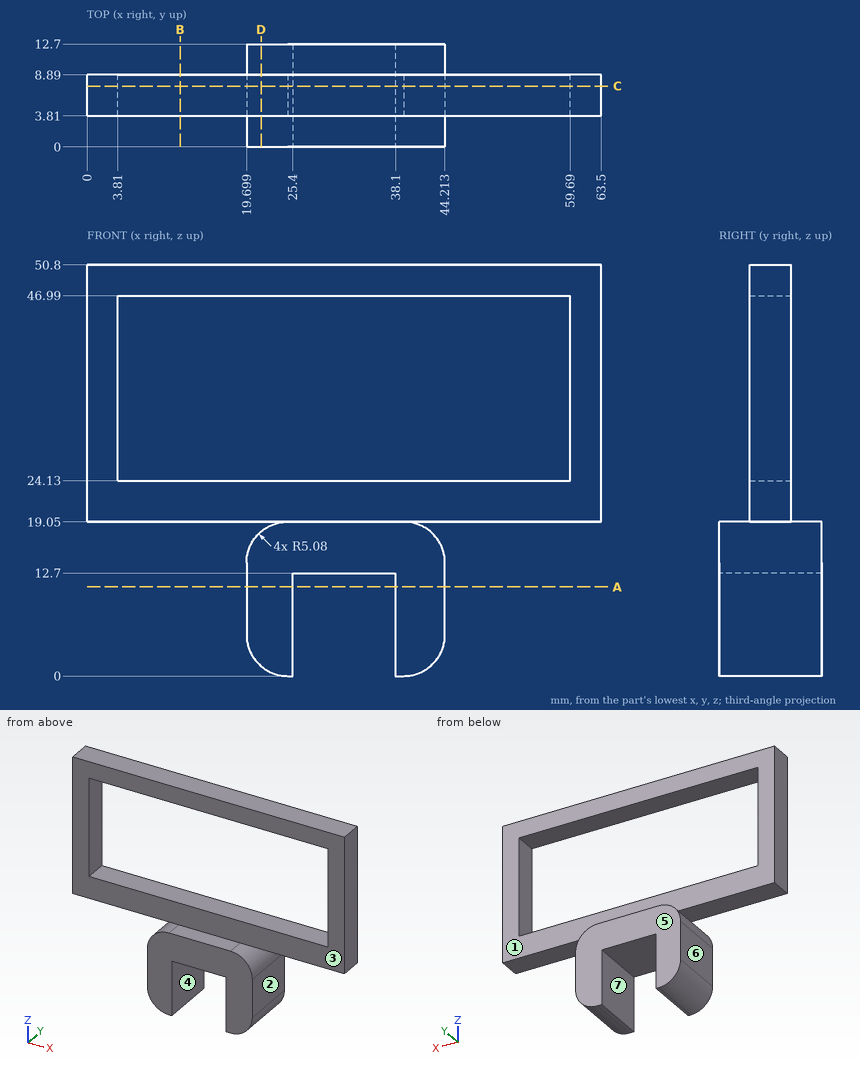
Answer from the drawing. Dimensions are ordinates in mm from the lowest x, y and z of the part. A direction names the side the tool comes from. Give positions to 0.01 mm unless a question says otherwise; leave off trailing zeros. Order: outer loops, then holes, each group sorted by start corner. A loop starts at its lowest first (then second) coordinate and runs counter-clockwise, first axis right, second up. Notation, with made-up numbers: (88.25, 5) -> (98.25, 5) arc R26 ccw to (98.25, 19) -> close; hole circle Ø11 at (10.25, 58). An arc over 180 degrees is marked (long way). Answer as a JSON object with one key per item and string values. Group by question number.
1. Flat-ended cylindrical pins translate along their axes: pin 1 Ø3 at (x, z) = (49.5, 44.5) entering from +Y (3 decimals); pin 2 Ø4 at (x, y) = (22.5, 6) entering from -Z; pin 3 Ø2 at (y, z) = (2, 9) entering from +X; pin 4 Ø4 at (y, z) = (6.5, 3.5) entering from -X. Find the tip coordinate at first contact, or state that the pin passes through.
2. Section B-B on x = 11.5 is taken. Determine the outline of the cut face in (y, z).
3. Section C-C on y = 7.5 is taken. Determine the outline of the cut face in (x, z).
4. Consider line 1 along Z through (x, y) = (54.5, 4); line 2 along X through (y, z) = (8.25, 33); line 3 along X through (y, z) = (1.5, 12). Determine where each line is inside the solid, lowest interval first. Write a range as [from, to].
5. Section A-A on z = 11 is taken. Determine the outline of the cut face in (x, y).
6. A tool of negligible diameter and unlimited length cuts with its end or side. For the marked faces 1, 2, 3 and 4, from which of +Z, -Z, +X, -X, +Y, -Y can it reach the whole face along a straight path? Write none if from no direction.
7. The mould has two halves that part along X. Classify the marked faces 5, 6 and 7: released by +X, released by -X, zero draft, split by the parting line, or undercut.
8. Section D-D on x = 21.5 is taken. Determine the outline of the cut face in (y, z), plus the area to 3 significant figures.
Result sheet:
{
 "1": {"pin 1": "passes through", "pin 2": "stops at z = 0.01", "pin 3": "stops at x = 44.21", "pin 4": "stops at x = 19.7"},
 "2": {"outline": "(3.81, 19.05) -> (8.89, 19.05) -> (8.89, 24.13) -> (3.81, 24.13) -> close; (3.81, 46.99) -> (8.89, 46.99) -> (8.89, 50.8) -> (3.81, 50.8) -> close"},
 "3": {"outline": "(0, 19.05) -> (24.78, 19.05) arc R5.08 ccw to (19.7, 13.97) -> (19.7, 5.08) arc R5.08 ccw to (24.78, 0) -> (25.4, 0) -> (25.4, 12.7) -> (38.1, 12.7) -> (38.1, 0) -> (39.13, 0) arc R5.08 ccw to (44.21, 5.08) -> (44.21, 13.97) arc R5.08 ccw to (39.13, 19.05) -> (63.5, 19.05) -> (63.5, 50.8) -> (0, 50.8) -> close; hole (3.81, 24.13) -> (59.69, 24.13) -> (59.69, 46.99) -> (3.81, 46.99) -> close"},
 "4": {"line 1": "z = [19.05, 24.13], [46.99, 50.8]", "line 2": "x = [0, 3.81], [59.69, 63.5]", "line 3": "x = [19.7, 25.4], [38.1, 44.21]"},
 "5": {"outline": "(19.7, 0) -> (25.4, 0) -> (25.4, 12.7) -> (19.7, 12.7) -> close; (38.1, 0) -> (44.21, 0) -> (44.21, 12.7) -> (38.1, 12.7) -> close"},
 "6": {"face 1": "+Z, +X, -X, +Y", "face 2": "-Z, +X, +Y, -Y", "face 3": "+Z, +X, -X, -Y", "face 4": "-Z, +Y, -Y"},
 "7": {"face 5": "zero draft", "face 6": "released by -X", "face 7": "undercut"},
 "8": {"outline": "(0, 1.2) -> (12.7, 1.2) -> (12.7, 17.85) -> (0, 17.85) -> close; (3.81, 19.05) -> (8.89, 19.05) -> (8.89, 24.13) -> (3.81, 24.13) -> close; (3.81, 46.99) -> (8.89, 46.99) -> (8.89, 50.8) -> (3.81, 50.8) -> close", "area": "257 mm^2"}
}
